Geometry check sheet. Reference: drawing and pictorial views, mm from the part's lowest x, y, z. Round coordinates to 2 decimals unless told otherwise and drop trailing zeros. Write each loop counter-clockwise with the first axis right and the second up, starting at its lowest first coordinate (ties: lowest second). Pieces come first, ordered by that corner, then holes. Notation, with made-up numbers: (19, -37.5) -> (50, -37.5) arc R19 ccw to (50, -20.5) -> close; hole circle Ø8 at (37, 32). An arc over 180 degrees is marked (long way). Answer as a JSON object with one key per item and string values. Group by question number.
(1) Gauge pin test, flat ends, axial feed: pin 1 Ø1 at (y, z) = (56, 2) entering from +X; pin 2 Ø2.5 at (x, z) = (95, 2.5) entering from -Y; pin 3 Ø1.5 at (y, z) = (47, 3) entering from -X; pin 4 Ø2 at (x, z) = (128, 3) entering from +Y. Record the tip position at first contact, or that the pin passes through.
(2) Sectioned sample at B-B on x = 13. Record the cut outline in (y, z), and give its area (3 significant figures).
(3) Sectioned sample at A-A on y = 95. Record the cut outline in (x, z), and give its area (3 significant figures).
(4) Scan lines: L1, parallel to Y at x = 92.5, z = 2.45; L2, parallel to Z at x = 95, y = 187.35; L3, parallel to Y at x = 171.5, z = 1.9. Record each from-to range of solid material in increasing order. Write a range as from..to.
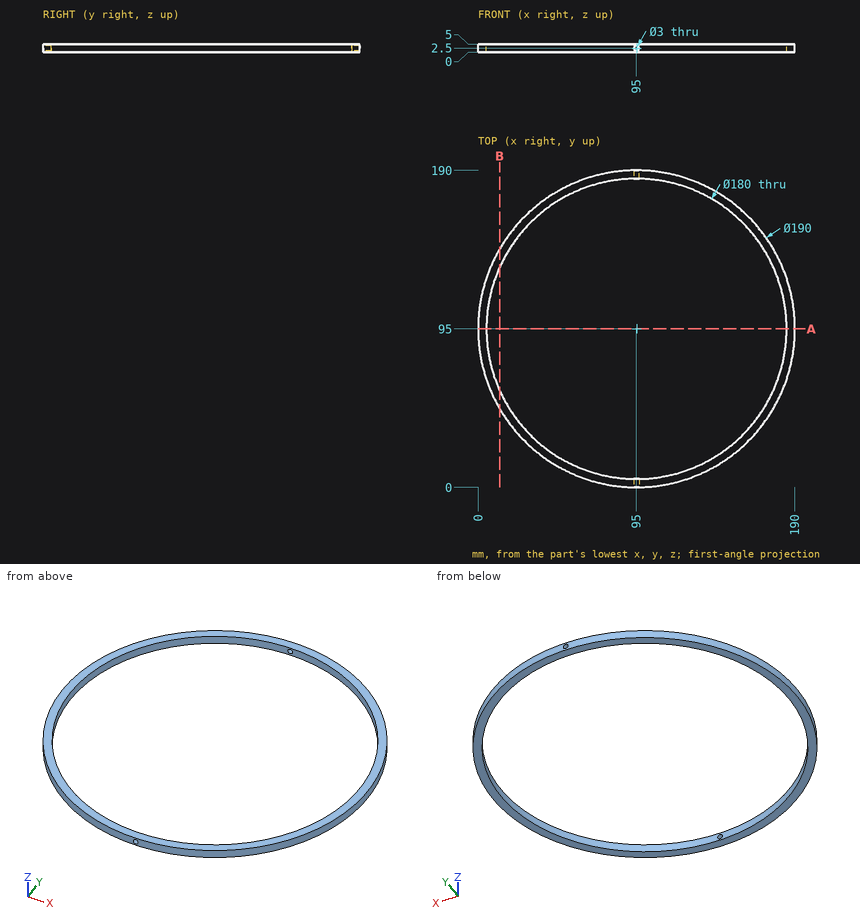
Computed values:
{
 "1": {"pin 1": "x = 181.85", "pin 2": "through", "pin 3": "x = 12.58", "pin 4": "y = 184.45"},
 "2": {"outline": "(47.03, 0) -> (57.91, 0) -> (57.91, 5) -> (47.03, 5) -> close; (132.09, 0) -> (142.97, 0) -> (142.97, 5) -> (132.09, 5) -> close", "area": "109 mm2"},
 "3": {"outline": "(0, 0) -> (5, 0) -> (5, 5) -> (0, 5) -> close; (185, 0) -> (190, 0) -> (190, 5) -> (185, 5) -> close", "area": "50.0 mm2"},
 "4": {"L1": "0.03..5.03, 184.97..189.97", "L2": "0..1, 4..5", "L3": "38.67..47.59, 142.41..151.33"}
}
